```python
from build123d import *

# Parameters (mm, degrees)
SKETCH_1_R          = 1.2
EXTRUDE_1_DEPTH     = 2
SKETCH_2_W          = 21
SKETCH_2_H          = 13.5
EXTRUDE_2_DEPTH     = 12
SKETCH_3_R          = 4
CUT_EXTRUDE_1_DEPTH = 4
SKETCH_4_W          = 19
SKETCH_4_H          = 4
EXTRUDE_3_DEPTH     = 3
SKETCH_5_R          = 6
EXTRUDE_4_DEPTH     = 5


with BuildPart() as part:
    # 草图1 → 凸台-拉伸1 (new body)
    with BuildSketch(Plane(origin=(0, 0, 0), x_dir=(1, 0, 0), z_dir=(0, 1, 0))):
        Polygon((10.5, 17.5), (13.5, 17.5), (13.5, -17.5), (-13.5, -17.5), (-13.5, 17.5), (-10.5, 17.5), (-10.5, 28.5), (10.5, 28.5), align=None)
        with Locations(Location((12.25, -11, 0), (0, 0, 270))):
            Circle(SKETCH_1_R, mode=Mode.SUBTRACT)
        with Locations(Location((12.25, 15.5, 0), (0, 0, 270))):
            Circle(SKETCH_1_R, mode=Mode.SUBTRACT)
        with Locations(Location((-12.25, 15.5, 0), (0, 0, 90))):
            Circle(SKETCH_1_R, mode=Mode.SUBTRACT)
        with Locations(Location((-12.25, -11, 0), (0, 0, 90))):
            Circle(SKETCH_1_R, mode=Mode.SUBTRACT)
    extrude(amount=EXTRUDE_1_DEPTH)

    # 草图2 → 凸台-拉伸2 (add)
    with BuildSketch(Plane.XZ):
        with Locations((0, -24.25)):
            Rectangle(SKETCH_2_W, SKETCH_2_H)
    extrude(amount=EXTRUDE_2_DEPTH)

    # 草图3 → 切除-拉伸1 (cut)
    with BuildSketch(Plane(origin=(0, 0, -31), x_dir=(-1, 0, 0), z_dir=(0, 0, -1))):
        with Locations((0, -6)):
            Circle(SKETCH_3_R)
    extrude(amount=-CUT_EXTRUDE_1_DEPTH, mode=Mode.SUBTRACT)

    # 草图4 → 凸台-拉伸3 (add)
    with BuildSketch(Plane.XZ):
        with Locations((0, 15.5)):
            Rectangle(SKETCH_4_W, SKETCH_4_H)
    extrude(amount=EXTRUDE_3_DEPTH)

    # 草图5 → 凸台-拉伸4 (add)
    with BuildSketch(Plane.XZ):
        with Locations(Location((-3.274170516, 1.847483042, 0), (0, 0, 270))):
            Circle(SKETCH_5_R)
    extrude(amount=EXTRUDE_4_DEPTH)


solid = part.part
```
Geometry: final body of the model. Coordinates: model frame, mm. A direction names the side the tool comes from. Give positions to 0.01 mm unless a question says otherwise; leave off trailing zeros. Loops run counter-clockwise (first coordinate to the right, second up) from the corner with the lowest first, then second, coordinate; pieces in that order, holes last. Notation, with made-up numbers: (39.5, 28.25) - (71.5, 28.25) arc R18 cw to (71.5, 62.25) - close; hole circle Ø2 at (-3.5, 50.25). An arc over 180 degrees is marked (long way). Answer as CSV lines item,"result". Start each with the question number.
(1) Mould query, pull axis X, two halves, no side actions, for faces 1 (the face through (0, 2, -6)), 2 (the face through (0, -6, -27)), 3 (the face through (11.08, 0.99, 10.74)), 4 (the face through (-3.01, -2.46, 7.84)). Classes: +X half, -X half, draft (parallel to the pull), parting line (faces both ways), or undercut.
(2) Pin query (flat end, axial travel): P1, Ø1.2, axis at x = -5, z = -29.5, coming from the +Y side; P2, Ø2, axis at x = -3.5, y = 1.5, coming from the -Z side; P3, Ø0.6, axis at x = 12, y = 1.5, coming from the -Z side; P4, Ø4, axis at x = 12.25, z = 11, coming from the +Y side. Return the tip coordinate at first contact, or that it passes through.
(3) Section query B-B (z = -15.5). Output: boundary loops of the cut face in (x, y).
(4) Section query A-A (x = 12.25). Output: boundary loops of the cut face in (y, z).
(5) Section query D-D (y = -6). Output: boundary loops of the cut face in (x, z), and give its area (4 significant figures).
(6) Reachability of faces 5 (the face through (0.867, -9.905, -29.028)), 6 (the face through (0, 0, -30)), 7 (the face through (12, 1, -17.5)), 8 (the face through (0, -6, -17.5)) from +Z, -Z, +X, -X, +Y, -Y: full face, straight path, thin tool, end or side. Return the list, or none.
(7) Section query C-C (x = 8). Output: boundary loops of the cut face in (y, z), and give its area (3 significant figures).
(8) Ray query, line 1 along Z through (x, y) = (-3, -2.25); line 2 along Z through (x, y) = (2.25, -0.25); line 3 along Z through (x, y) = (7, -2.25). Return the intervals inside material, ascending. Write a range as [from, to].
Worked answers:
1,face 1,"draft"
1,face 2,"undercut"
1,face 3,"undercut"
1,face 4,"parting line"
2,P1,"stops at y = 0"
2,P2,"stops at z = -28.5"
2,P3,"stops at z = -17.5"
2,P4,"stops at y = 2"
3,outline,"(-13.5, 0) - (-13.45, 0) - (-13.45, 2) - (-13.5, 2) - close; (-11.05, 0) - (11.05, 0) - (11.05, 2) - (-11.05, 2) - close; (13.45, 0) - (13.5, 0) - (13.5, 2) - (13.45, 2) - close"
4,outline,"(0, -17.5) - (2, -17.5) - (2, -16.7) - (0, -16.7) - close; (0, -14.3) - (2, -14.3) - (2, 9.8) - (0, 9.8) - close; (0, 12.2) - (2, 12.2) - (2, 17.5) - (0, 17.5) - close"
5,outline,"(-10.5, -31) - (-4, -31) - (-4, -27) - (4, -27) - (4, -31) - (10.5, -31) - (10.5, -17.5) - (-10.5, -17.5) - close"
5,area,"251.5 mm^2"
6,face 5,"-Z"
6,face 6,"-Z, +X, -X, +Y"
6,face 7,"-Z, +X, +Y, -Y"
6,face 8,"+X, -X, -Y"
7,outline,"(-12, -31) - (0, -31) - (0, -28.5) - (2, -28.5) - (2, 17.5) - (-3, 17.5) - (-3, 13.5) - (0, 13.5) - (0, -17.5) - (-12, -17.5) - close"
7,area,"266 mm^2"
8,line 1,"z = [-31, -17.5], [-4.15, 7.84], [13.5, 17.5]"
8,line 2,"z = [-31, -17.5], [-0.49, 4.19], [13.5, 17.5]"
8,line 3,"z = [-31, -17.5], [13.5, 17.5]"
